Autodesk Inventor part; units mm, degrees
ref_plane "YZ Plane" through (0, 0, 0) normal (1, 0, 0) x (0, 1, 0)
ref_plane "XZ Plane" through (0, 0, 0) normal (0, 1, 0) x (-1, 0, 0)
ref_plane "XY Plane" through (0, 0, 0) normal (0, 0, 1) x (1, 0, 0)
sketch "Sketch1" plane through (0, 0, 0) normal (0, 1, 0) x (-1, 0, 0)
  line L0 (-9, 6) -> (-9, -6)
  line L1 (-9, -6) -> (9, -6)
  line L2 (9, -6) -> (9, 6)
  line L3 (9, 6) -> (-9, 6)
  line L4 (-9, 6) -> (9, -6) construction
  line L5 (-9, -6) -> (9, 6) construction
  point P0 (0, 0)
  dimension "d0" = 12
  dimension "d1" = 18
extrude "Extrusion1" add sketch "Sketch1" along normal blind 12
sketch "Sketch2" plane through (0, 12, 0) normal (0, 1, 0) x (1, 0, 0)
  line L0 (10.5, -7.5) -> (10.5, 7.5)
  line L1 (10.5, 7.5) -> (-10.5, 7.5)
  line L2 (-10.5, 7.5) -> (-10.5, -7.5)
  line L3 (-10.5, -7.5) -> (10.5, -7.5)
  line L4 (10.5, -7.5) -> (-10.5, 7.5) construction
  line L5 (10.5, 7.5) -> (-10.5, -7.5) construction
  point P0 (0, 0)
  dimension "d4" = 15
  dimension "d5" = 21
extrude "Extrusion2" add sketch "Sketch2" along normal blind 2
chamfer "Chamfer1" distance 1.8 distance2 1.2 1 edges at (10.5, 14, 0) measured on face at (-3.5, 14, -2.5)
chamfer "Chamfer2" distance 1.8 distance2 1.2 1 edges at (-0.9, 14, 7.5) measured on face at (-4.1, 14, -2.5)
chamfer "Chamfer3" distance 1.8 distance2 1.2 1 edges at (-10.5, 14, -0.9) measured on face at (-4.1, 14, -3.1)
chamfer "Chamfer4" distance 1.8 distance2 1.2 1 edges at (0, 14, -7.5) measured on face at (2.9, 14, 1.3)
sketch "Sketch3" plane through (0, 14, 0) normal (0, 1, 0) x (1, 0, 0)
  line L0 (-8.7, 5.7) -> (8.7, 5.7)
  line L1 (-8.7, -5.7) -> (-8.7, 5.7)
  line L2 (8.7, -5.7) -> (-8.7, -5.7)
  line L3 (8.7, 5.7) -> (8.7, -5.7)
  point P0 (0, 0)
extrude "Extrusion3" add sketch "Sketch3" along normal blind 3
sketch "Sketch4" plane through (-8.7, 14, 5.7) normal (0, 0, 1) x (1, 0, 0)
  line L0 (17.4, 0) -> (0, 0)
  line L1 (17.4, 0) -> (17.4, 3)
  line L2 (0, 3) -> (17.4, 3)
  line L3 (0, 0) -> (0, 3)
  line L4 (17.4, 0) -> (17.4, 3)
  line L5 (17.4, 3) -> (0, 3)
  line L6 (0, 3) -> (0, 0)
  line L7 (0, 0) -> (17.4, 0)
  line L8 (17.4, 0) -> (16.7, 0)
  line L9 (17.4, 0) -> (0, 0)
  line L10 (16.7, 0) -> (16.7, 3)
  line L11 (0, 3) -> (17.4, 3)
  arc A0 (0, 0) -> (16.7, 3) centre (-4.649, 73.861) ccw
  arc A1 (17.4, 0) -> (16.7, 3) centre (10.8425, 0.0516) ccw
  point P0 (8.7, -14)
  dimension "d24" = 0.7
extrude "Extrusion4" cut sketch "Sketch4" against normal through all contours A1 L2 L1 | A0 L3 L2
sketch "Sketch5" plane through (0, 0, 0) normal (0, -1, 0) x (1, 0, 0)
  line L0 (0.5, -3) -> (0.5, 3)
  line L1 (0.5, 3) -> (-0.5, 3)
  line L2 (-0.5, 3) -> (-0.5, -3)
  line L3 (-0.5, -3) -> (0.5, -3)
  line L4 (0.5, -3) -> (-0.5, 3) construction
  line L5 (0.5, 3) -> (-0.5, -3) construction
  line L6 (0, 0) -> (-7, 0)
  line L7 (0, 0) -> (7, 0)
  line L8 (-6.5, -3) -> (-6.5, 3)
  line L9 (-6.5, 3) -> (-7.5, 3)
  line L10 (-7.5, 3) -> (-7.5, -3)
  line L11 (-7.5, -3) -> (-6.5, -3)
  line L12 (-6.5, -3) -> (-7.5, 3) construction
  line L13 (-6.5, 3) -> (-7.5, -3) construction
  line L14 (7.5, -3) -> (7.5, 3)
  line L15 (7.5, 3) -> (6.5, 3)
  line L16 (6.5, 3) -> (6.5, -3)
  line L17 (6.5, -3) -> (7.5, -3)
  line L18 (7.5, -3) -> (6.5, 3) construction
  line L19 (7.5, 3) -> (6.5, -3) construction
  dimension "d27" = 6
  dimension "d28" = 1
  dimension "d29" = 7
  dimension "d30" = 7
  dimension "d31" = 1
  dimension "d32" = 1
  dimension "d41" = 6
  dimension "d42" = 6
extrude "Extrusion5" add sketch "Sketch5" along normal blind 8
chamfer "Chamfer5" distance 1.5 angle 45 6 edges at (7, -8, -3) (7, -8, 3) (0, -8, 3) (-7, -8, 3) (-7, -8, -3) (0, -8, -3)
properties part number "Toggle switch"
Part model, mm, in its own coordinate system. A direction names the side the tool comes from. Round coordinates to 2 decimals unless told otherwise and drop trailing zeros. Loops run counter-clockwise (first coordinate to the right, second up) from the corner with the lowest first, then second, coordinate; pieces in that order, holes last.
1. Slice it at B-B (z = -0.25). Give the cut face in (x, y).
Solutions:
outline: (-10.5, 12) - (-9, 12) - (-9, 0) - (-7.5, 0) - (-7.5, -8) - (-6.5, -8) - (-6.5, 0) - (-0.5, 0) - (-0.5, -8) - (0.5, -8) - (0.5, 0) - (6.5, 0) - (6.5, -8) - (7.5, -8) - (7.5, 0) - (9, 0) - (9, 12) - (10.5, 12) - (10.5, 12.8) - (8.7, 14) arc R6.56 ccw to (8, 17) arc R74.01 cw to (-8.7, 14) - (-10.5, 12.8) - close
2. Two-plate mould, pull along X, no slides. Class faces 6 (the face through (-7, -8, 0)), 7 (the face through (-9, 6, 0)), 8 (the face through (7.5, -4, 0)), 9 (the face through (-0.5, -4, 0)): pulls with the +X half, pulls with the -X half, needs draft (parallel to the pull), parting line crosses it, or undercut.
Solutions:
face 6: needs draft
face 7: pulls with the -X half
face 8: pulls with the +X half
face 9: undercut
3. Slice it at C-C (x = 2.5). Give the cut face in (y, z), and give its area (3 significant figures).
Solutions:
outline: (0, -6) - (12, -6) - (12, -7.5) - (12.8, -7.5) - (14, -5.7) - (15.57, -5.7) - (15.57, 5.7) - (14, 5.7) - (12.8, 7.5) - (12, 7.5) - (12, 6) - (0, 6) - close
area: 190 mm2
4. 3-axis set-ups, long thin cutter, end or side, ignore diameter. For faces 1 (the face through (-7.5, -4, 0)), 2 (the face through (-7, -3, 3)), 3 (the face through (4, 15, 5.7)), 4 (the face through (9, 6, 0)), 5 (the face through (-7, -3, -3)): which of +Z, -Z, +X, -X, +Y, -Y reach the whole face in a straight line?
Solutions:
face 1: +Z, -Z, -X, -Y
face 2: +Z, +X, -X, -Y
face 3: +Z, +X, -X, +Y
face 4: +Z, -Z, +X, -Y
face 5: -Z, +X, -X, -Y
5. Slice it at D-D (z = -2.25). Give the cut face in (x, y), and give its area (3 significant figures).
Solutions:
outline: (-10.5, 12) - (-9, 12) - (-9, 0) - (-7.5, 0) - (-7.5, -7.25) - (-6.5, -7.25) - (-6.5, 0) - (-0.5, 0) - (-0.5, -7.25) - (0.5, -7.25) - (0.5, 0) - (6.5, 0) - (6.5, -7.25) - (7.5, -7.25) - (7.5, 0) - (9, 0) - (9, 12) - (10.5, 12) - (10.5, 12.8) - (8.7, 14) arc R6.56 ccw to (8, 17) arc R74.01 cw to (-8.7, 14) - (-10.5, 12.8) - close
area: 299 mm2
6. Drill centre lines: line 1 along X through (y, z) = (-3.75, -2); line 2 along X through (y, z) = (3.75, -2.5); line 3 along Z through (x, y) = (-8, 10.75). Where is each one in solid material? Low to high.
Solutions:
line 1: x = -7.5 to -6.5, -0.5 to 0.5, 6.5 to 7.5
line 2: x = -9 to 9
line 3: z = -6 to 6
7. Slice it at A-A (y = -2). Give the cut face in (x, z).
Solutions:
outline: (-7.5, -3) - (-6.5, -3) - (-6.5, 3) - (-7.5, 3) - close; (-0.5, -3) - (0.5, -3) - (0.5, 3) - (-0.5, 3) - close; (6.5, -3) - (7.5, -3) - (7.5, 3) - (6.5, 3) - close
8. Flat gauge pins, fed straight in: pin 1 (1.5 mm diameter, centred on x = 0.5, y = -4, fed in from -Z); pin 2 (8 mm diameter, centred on x = -1, y = -1.5, fed in from -Z); pin 3 (6.5 mm diameter, centred on y = -5.5, z = 0, fed in from +X). Where does each tip first touch, or does it go through?
Solutions:
pin 1: stops at z = -3
pin 2: stops at z = -6
pin 3: stops at x = 7.5
